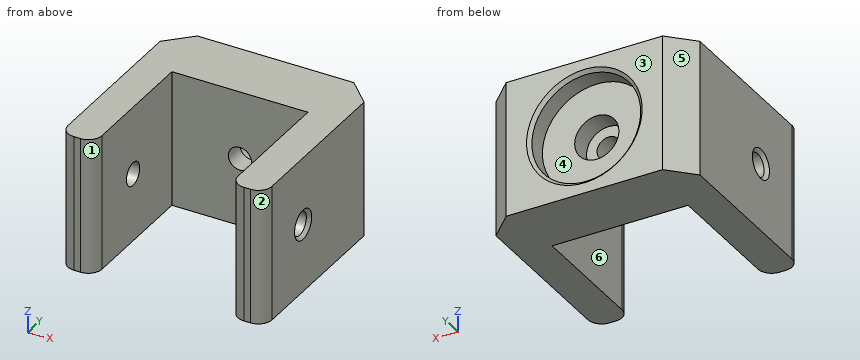
Autodesk Inventor part; units mm, degrees
ref_plane "YZ Plane" through (0, 0, 0) normal (1, 0, 0) x (0, 1, 0)
ref_plane "XZ Plane" through (0, 0, 0) normal (0, 1, 0) x (-1, 0, 0)
ref_plane "XY Plane" through (0, 0, 0) normal (0, 0, 1) x (1, 0, 0)
sketch "Sketch1" plane through (0, 0, 0) normal (0, 1, 0) x (-1, 0, 0)
  circle A0 centre (0, 0) radius 8
  line L0 (15, -10) -> (-15, -10)
  line L1 (-15, -10) -> (-15, 10)
  line L2 (-15, 10) -> (15, 10)
  line L3 (15, 10) -> (15, -10)
  point P0 (-15, 0)
  point P1 (0, -10)
  dimension "d0" = 30
  dimension "d1" = 16
  dimension "d2" = 20
extrude "Extrusion1" add sketch "Sketch1" against normal blind 6 contours A0 | L0 L1 L2 L3
extrude "Extrusion2" add sketch "Sketch1" along normal blind 3.2
hole "Hole1" at (0, 0, 0) direction (0, -1, 0) diameter 3.4 depth 10 counterbore diameter 6.5 counterbore depth 3.05
sketch "Sketch2" plane through (0, -6, 0) normal (0, -1, 0) x (1, 0, 0)
  circle A0 centre (0, 0) radius 1.7
  line L0 (15, 10) -> (-15, 10)
  line L1 (-15, 10) -> (-15, -10)
  line L2 (-15, -10) -> (15, -10)
  line L3 (15, -10) -> (15, 10)
  line L4 (-15, 10) -> (-15, -10)
  line L5 (-15, 10) -> (-10, 10)
  line L6 (-10, 10) -> (-10, -10)
  line L7 (-10, -10) -> (-15, -10)
  line L8 (-15, -10) -> (-15, 10)
  line L9 (-15, -10) -> (15, -10)
  line L10 (15, 10) -> (-15, 10)
  line L11 (15, -10) -> (10, -10)
  line L12 (10, -10) -> (10, 10)
  line L13 (10, 10) -> (15, 10)
  line L14 (15, 10) -> (15, -10)
  point P0 (10, 10)
  dimension "d14" = 5
  dimension "d15" = 5
extrude "Extrusion3" add sketch "Sketch2" along normal blind 20 contours L3 L2 L12 L0 | L6 L2 L1 L0
chamfer "Chamfer1" distance 3.5 angle 45 2 edges at (15, 3.2, 0) (-15, 3.2, 0)
fillet "Fillet1" radius 2 4 edges at (-15, -26, 0) (-10, -26, 0) (10, -26, 0) (15, -26, 0)
sketch "Sketch3" plane through (15, -0.3, 10) normal (1, 0, 0) x (0, 0, -1)
  line L0 (20, -23.7) -> (0, -23.7)
  line L1 (20, -5.7) -> (20, -23.7)
  line L2 (0, -5.7) -> (20, -5.7)
  line L3 (0, -5.7) -> (0, -23.7)
  line L4 (0, -25.7) -> (20, -25.7)
  line L5 (20, -25.7) -> (0, -25.7)
  line L6 (0, -5.7) -> (0, -23.7)
  line L7 (0, -25.7) -> (0, -5.7)
  point P0 (10, 0.3)
  point P1 (0, -15.7)
  point P2 (10, -25.7)
  point P3 (10, -25.7)
  point P4 (10, -15.7)
hole "Hole2" at (15, -16, 0) direction (-1, 0, 0) diameter 3.4 end through all
chamfer "Chamfer2" distance 0.5 angle 45 3 edges at (8, 3.2, 0) (15, -16, 1.7) (-15, -16, 1.7)
equation "\"d15\" = d14"
properties part number "Magnet Mount"
Verification items for the finished model (mm, model axes). Face numbers are marked on the shaded views. A direction names the side the tool comes from. Give positions to 0.01 mm unless a question says otherwise; leave off trailing zeros. Write each loop counter-clockwise with the first axis right and the second up, starting at its lowest first coordinate (ties: lowest second). Pieces come first, ordered by that corner, then holes. Notation, with made-up numbers: (29, 87) -> (64, 87) arc R17 cw to (64, 94) -> close; hole circle Ø3 at (79, 7). An arc over 180 degrees is marked (long way). Use CSV: the item, a comma, the result in double quotes.
(1) Go/stop test with flat-tipped pins: pin 1 (10 mm diameter, centred on x = -1.5, z = -3.5, fed in from -Y); pin 2 (7 mm diameter, centred on x = -1, z = -1, fed in from +Y); pin 3 (8 mm diameter, centred on x = -0.5, z = -4, fed in from +Y). Record where each tip stops, or that it passes through.
Derived:
pin 1,"stops at y = -6"
pin 2,"stops at y = 0"
pin 3,"stops at y = 2.73"
(2) Sectioned sample at A-A (x = 0). Record the cut outline in (y, z), plus the area to 3 significant figures.
Derived:
outline,"(-6, -10) -> (3.2, -10) -> (3.2, -8.5) -> (2.7, -8) -> (0, -8) -> (0, -3.25) -> (-3.05, -3.25) -> (-3.05, -1.7) -> (-6, -1.7) -> close; (-6, 1.7) -> (-3.05, 1.7) -> (-3.05, 3.25) -> (0, 3.25) -> (0, 8) -> (2.7, 8) -> (3.2, 8.5) -> (3.2, 10) -> (-6, 10) -> close"
area,"103 mm^2"
(3) Sectioned sample at B-B (y = -16). Record the cut outline in (x, z).
Derived:
outline,"(-15, -10) -> (-10, -10) -> (-10, -1.7) -> (-14.5, -1.7) -> (-15, -2.2) -> close; (-15, 2.2) -> (-14.5, 1.7) -> (-10, 1.7) -> (-10, 10) -> (-15, 10) -> close; (10, -10) -> (15, -10) -> (15, -2.2) -> (14.5, -1.7) -> (10, -1.7) -> close; (10, 1.7) -> (14.5, 1.7) -> (15, 2.2) -> (15, 10) -> (10, 10) -> close"
(4) Sectioned sample at C-C (y = -21.75). Record the cut outline in (x, z).
Derived:
outline,"(-15, -10) -> (-10, -10) -> (-10, 10) -> (-15, 10) -> close; (10, -10) -> (15, -10) -> (15, 10) -> (10, 10) -> close"
(5) Release check for a two-part mould opening along X. For the marked faces 1, 2 and 3 record: +X half, -X half, draft (parallel to the pull), parting line (faces both ways), or undercut.
Derived:
face 1,"undercut"
face 2,"+X half"
face 3,"draft"
(6) Sectioned sample at D-D (x = -12.5). Record the cut outline in (y, z), plus the area to 3 significant figures.
Derived:
outline,"(-26, -10) -> (2.2, -10) -> (2.2, 10) -> (-26, 10) -> close; hole circle Ø3.4 at (-16, 0)"
area,"555 mm^2"
(7) Material ranges on L1, parallel to Z at x = 11.7, y = -16; L2, parallel to X at y = -1.25, z = 0; L3, parallel to X at y = -16, z = -8, recorded low to high.
Derived:
L1,"z = -10 to -1.7, 1.7 to 10"
L2,"x = -15 to -3.25, 3.25 to 15"
L3,"x = -15 to -10, 10 to 15"
(8) Set-up check for the marked faces 4, 5 and 6: record each of +Z, -Z, +X, -X, +Y, -Y from which the full face is reachable in a straight line by a thin tool's end or side.
Derived:
face 4,"+Y"
face 5,"+Z, -Z, -X, +Y"
face 6,"+Z, -Z, -Y"
